Part model, mm, in its own coordinate system. Face numbers are marked on the shaded views. A direction names the side the tool comes from. Coordinates: 2 decimals unless noted, no trailing zeros. Write each loop counter-clockwise with the first axis right and the second up, starting at its lowest first coordinate (ties: lowest second). Pieces come first, ordered by that corner, then holes. Notation, with made-up numbers: (85.5, -10.5) -> (128.5, -10.5) arc R26 cw to (128.5, 9.5) -> close; hole circle Ø7 at (39, 1.25). An arc over 180 degrees is marked (long way). One line per question, with ' | ' between items. Start each with the question number.
Item 1: Saw through at C-C (x = -7). List the corners of the cut face in (y, z), and give its area (3 significant figures).
Item 2: Saw through at B-B (y = 18). List the corners of the cut face in (x, z), and give its area (3 significant figures).
Item 3: 3-axis set-ups, long thin cutter, end or side, ignore diameter. For the marked faces 5 and 6: which of +Z, -Z, +X, -X, +Y, -Y reach the whole face in a straight line?
Item 4: Pin check, flat tip, straight feed: pin 1 (9 mm diameter, centred on x = 3, z = 3, fed in from -Y). Stop position of the tip, or through.
Item 5: Two-plate mould, pull along X, no slides. Class the marked faces 1, 2, 3 and 4: pulls with the +X half, pulls with the -X half, needs draft (parallel to the pull), parting line crosses it, or undercut.
Item 6: Saw through at A-A (z = -11). List the corners of the cut face in (x, y).
Item 7: Probe probe 1 along Z at (x, y) = (13.5, 3); probe 2 along Y at (x, z) = (3.5, -11). List the from-to ranges inside material, lowest first. Write a range as [from, to].
Autodesk Inventor part; units mm, degrees
ref_plane "YZ Plane" through (0, 0, 0) normal (1, 0, 0) x (0, 1, 0)
ref_plane "XZ Plane" through (0, 0, 0) normal (0, 1, 0) x (-1, 0, 0)
ref_plane "XY Plane" through (0, 0, 0) normal (0, 0, 1) x (1, 0, 0)
sketch "Sketch1" plane through (0, 0, 0) normal (0, 1, 0) x (-1, 0, 0)
  line L0 (0, -24.5) -> (0, 24.5) construction
  line L1 (-24.5, 0) -> (24.5, 0) construction
  line L2 (17.5, 17.5) -> (-17.5, 17.5)
  line L3 (-17.5, 17.5) -> (-17.5, -17.5)
  line L4 (-17.5, -17.5) -> (17.5, -17.5)
  line L5 (17.5, -17.5) -> (17.5, 17.5)
  line L6 (15, 15) -> (-15, 15)
  line L7 (-15, 15) -> (-15, -15)
  line L8 (-15, -15) -> (15, -15)
  line L9 (15, -15) -> (15, 15)
  point P0 (0, 0)
  dimension "d0" = 35
  dimension "d1" = 35
  dimension "d2" = 30
  dimension "d3" = 30
extrude "Extrusion1" add sketch "Sketch1" along normal blind 30
sketch "Sketch2" plane through (0, 30, 0) normal (0, 1, 0) x (1, 0, 0)
  line L0 (-17.5, 17.5) -> (-17.5, -17.5)
  line L1 (-17.5, -17.5) -> (17.5, -17.5)
  line L2 (17.5, -17.5) -> (17.5, 17.5)
  line L3 (17.5, 17.5) -> (-17.5, 17.5)
  point P0 (0, 0)
extrude "Extrusion2" add sketch "Sketch2" along normal blind 2
properties part number "UG-752-30x30x32mm" material "Glass"
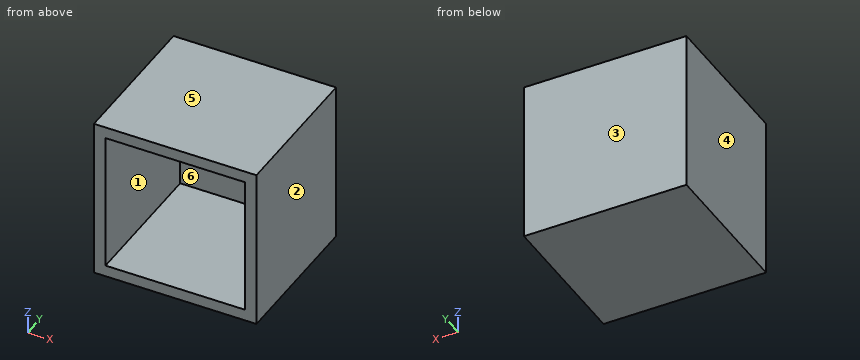
From the geometry:
1) outline: (0, -17.5) -> (32, -17.5) -> (32, 17.5) -> (0, 17.5) -> (0, 15) -> (30, 15) -> (30, -15) -> (0, -15) -> close | area: 220 mm2
2) outline: (-17.5, -17.5) -> (17.5, -17.5) -> (17.5, 17.5) -> (-17.5, 17.5) -> close; hole (-15, -15) -> (15, -15) -> (15, 15) -> (-15, 15) -> close | area: 325 mm2
3) face 5: +Z, +X, -X, +Y, -Y | face 6: -Y
4) pin 1: y = 30
5) face 1: undercut | face 2: pulls with the +X half | face 3: needs draft | face 4: pulls with the -X half
6) outline: (-17.5, 0) -> (-15, 0) -> (-15, 30) -> (15, 30) -> (15, 0) -> (17.5, 0) -> (17.5, 32) -> (-17.5, 32) -> close
7) probe 1: [-17.5, -15], [15, 17.5] | probe 2: [30, 32]
